from build123d import *

# Parameters (mm, degrees)
F0_W     = 59.69
F0_H     = 3
F1_DEPTH = 514.2
F3_DEPTH = 564.2
F4_SIZE  = 15


with BuildPart() as f1:
    # F0 (on Front) → F1 (new body)
    with BuildSketch(Plane.XZ):
        with Locations((29.845, 1.5)):
            Rectangle(F0_W, F0_H)
    extrude(amount=F1_DEPTH)

    # F2 (on face) → F3 (join)
    with BuildSketch(Plane(origin=(0, 0, 0), x_dir=(-1, 0, 0), z_dir=(0, 1, 0))):
        Polygon((-97.79, 0), (-59.69, 0), (-59.69, 3), (-59.69, 4), (-97.79, 4), (-97.79, 1.197734), align=None)
        Polygon((0, 4), (0, 3), (0, 0), (38.1, 0), (38.1, 4), align=None)
    extrude(amount=-F3_DEPTH)

    # F4
    f4_edges = [f1.edges().sort_by_distance(p)[0] for p in [
        (97.79, 0, 2),
        (-38.1, 0, 2),
    ]]
    chamfer(f4_edges, length=F4_SIZE)


solid = f1.part
Here's how the part is built. I have some questions about the finished solid (model axes, mm). Give positions to 0.01 mm unless a question says otherwise; leave off trailing zeros. Order: outer loops, then holes, each group sorted by start corner. A loop starts at its lowest first (then second) coordinate and runs counter-clockwise, first axis right, second up. Notation, with made-up numbers: (-11, -29.5) -> (38, -29.5) arc R28 cw to (38, -7.5) -> close; hole circle Ø8 at (-18.5, 84.25). An arc over 180 degrees is marked (long way). One line per item, written item: value. Start each with the question number.
1. Imagine slicing it at C-C, the plane x = 50. List the corners of the cut face in (y, z) for me, plus the area to 3 significant figures.
2. Imagine slicing it at A-A, the plane y = -341. List the corners of the cut face in (x, z) for me.
3. I need wall thicknesses on probe 1 along X at (y, z) = (-383.5, 3.7); probe 2 along Z at (x, y) = (59, -341); probe 3 along Y at (x, z) = (52, 2.15). Which ranges of each line are inside material? Lowest first, please. Write a range as from..to.
4. Imagine slicing it at B-B, the plane z = 1.95. List the corners of the cut face in (x, y) for me.
5. We'd pull the mould along X, two halves only. Please class faces 1 (the face through (-30.7, -7.6, 2)), 2 (the face through (29, -254, 3)), 3 (the face through (31, -278, 0)): released by +X, released by -X, zero draft, split by the parting line, or undercut.
6. Will these pins go through, and if not, where does the flat tip stop? pin 1 Ø6 at (x, y) = (36.5, -285.5) entering from +Z; pin 2 Ø1.5 at (x, z) = (39, 1.5) entering from -Y.
Values follow:
1. outline: (-514.2, 0) -> (0, 0) -> (0, 3) -> (-514.2, 3) -> close
1. area: 1,540 mm2
2. outline: (-38.1, 0) -> (97.79, 0) -> (97.79, 4) -> (59.69, 4) -> (59.69, 3) -> (0, 3) -> (0, 4) -> (-38.1, 4) -> close
3. probe 1: x = -38.1..0, 59.69..97.79
3. probe 2: z = 0..3
3. probe 3: y = -514.2..0
4. outline: (-38.1, -564.2) -> (0, -564.2) -> (0, -514.2) -> (59.69, -514.2) -> (59.69, -564.2) -> (97.79, -564.2) -> (97.79, -15) -> (82.79, 0) -> (-23.1, 0) -> (-38.1, -15) -> close
5. face 1: released by -X
5. face 2: undercut
5. face 3: zero draft
6. pin 1: stops at z = 3
6. pin 2: stops at y = -514.2
